Check sheet for the modelled part. Datum: model origin and axes. Units: mm. A direction names the side the tool comes from. Round coordinates to 2 decimals unless told otherwise and drop trailing zeros. Loops run counter-clockwise (first coordinate to the right, second up) from the corner with the lowest first, then second, coordinate; pieces in that order, holes last. Notation, with made-up numbers: M -0.75,54 L 12.25,54 A37 ccw 12.25,93 Z; hole C 67,-36.75 d10. An arc over 180 degrees is marked long. Write item = value, one per line. Start each with the question number.
(1) Cross-section at B-B on y = -45. Record the boundary of the cut face in (x, z), plus the area to 3 significant figures.
(2) Mould release check, pull along Y, two halves, no side actions. Record for faces 3 (the face through (-2, -36.282, 4)), 4 (the face through (-6, -26, 0)): pulls with the +Y half, pulls with the -Y half, needs draft (parallel to the pull), parting line crosses it, or undercut.
(3) Go/stop test with flat-tipped pins: P1, Ø6, axis at y = -50.5, z = -3, coming from the -X side; P2, Ø3, axis at x = -3, y = -42, coming from the -Z side; P3, Ø8, axis at x = -1.5, y = -39, coming from the -Z side. Record where each tip stops, or that it passes through.
(4) Cross-section at D-D on z = -5. Record the boundary of the cut face in (x, y), plus the area to 3 significant figures.
(5) Cross-section at C-C on z = -3. Record the boundary of the cut face in (x, y), plus the area to 3 significant figures.
(6) Scan lines: L1, parallel to Y at x = -10, z = -3; L2, parallel to Z at x = -13.5, y = -28; L3, parallel to X at y = -38.5, z = -3.75. Record each from-to range of solid material in increasing order. Write a range as from..to.
(7) Cross-section at A-A on z = 1. Record the boundary of the cut face in (x, y), plus the area to 3 significant figures.
(8) Set-up check for faces 1 (the face through (-6, -57.205, 0)), 2 (the face through (-11.766, -46.597, 1.22)): record each of +Z, -Z, +X, -X, +Y, -Y from which the full face is reachable in a straight line by a thin tool's end or side.
from build123d import *

# Parameters (mm, degrees)
SKETCH1_R      = 8.636
EXTRUDE1_DEPTH = 7.366
FILLET1_R      = 1.27
SKETCH2_W      = 6.080205461
SKETCH2_H      = 2.724463649
SKETCH3_R      = 5.626834032
EXTRUDE2_DEPTH = 20.922880412


with BuildPart() as part:
    # Sketch1 → Extrude1 (new body)
    with BuildSketch(Plane.XY):
        with Locations((-6.272807724, -26.314359982)):
            Circle(SKETCH1_R)
    extrude(amount=EXTRUDE1_DEPTH)

    # Fillet1
    fillet1_edges = [part.edges().sort_by_distance(p)[0] for p in [
        (-14.908807724, -26.314359982, 7.366),
    ]]
    fillet(fillet1_edges, radius=FILLET1_R)

    # Sketch2 → Revolve1 (revolve)
    with BuildSketch(Plane.XY, mode=Mode.PRIVATE) as revolve1_sk:
        with Locations((-9.312910455, -34.919678092)):
            Rectangle(SKETCH2_W, SKETCH2_H)
    revolve(revolve1_sk.sketch.rotate(Axis((-6.272807724, -33.557446268, 0), (0, -1, 0)), 270), axis=Axis((-6.272807724, -33.557446268, 0), (0, -1, 0)))

    # Sketch3 → Extrude2 (add)
    with BuildSketch(Plane.XZ.offset(36.281909917)):
        with Locations(Location((-6.272807724, 0, 0), (0, 0, 270))):
            Circle(SKETCH3_R)
    extrude(amount=EXTRUDE2_DEPTH)


solid = part.part
Result:
q1.outline = C -6.27,0 d11.25
q1.area = 99.5 mm^2
q2.face_3 = pulls with the -Y half
q2.face_4 = needs draft
q3.P1 = -11.9
q3.P2 = -5.34
q3.P3 = -5.8
q4.outline = M -9.73,-36.28 L -8.85,-36.28 L -8.85,-57.2 L -3.69,-57.2 L -3.69,-36.28 L -2.81,-36.28 L -2.81,-33.56 L -9.73,-33.56 Z
q4.area = 127 mm^2
q5.outline = M -11.56,-36.28 L -11.03,-36.28 L -11.03,-57.2 L -1.51,-57.2 L -1.51,-36.28 L -0.98,-36.28 L -0.98,-33.56 L -11.56,-33.56 Z
q5.area = 228 mm^2
q6.L1 = -57.2..-33.56
q6.L2 = 0..7.36
q6.L3 = -10.47..-2.08
q7.outline = M -12.27,-36.28 L -11.81,-36.28 L -11.81,-57.2 L -0.74,-57.2 L -0.74,-36.28 L -0.28,-36.28 L -0.28,-33.56 L -1.57,-33.56 A8.64 ccw long -10.98,-33.56 L -12.27,-33.56 Z
q7.area = 490 mm^2
q8.face_1 = +Z, -Z, +X, -X, -Y
q8.face_2 = -Y
